The drawing under review shows one solid part. Ordinate dimensions are in mm from its lowest x, y, z. A direction names the side the tool comes from. Give positions to 0.01 mm unless a question says otherwise; leave off trailing zeros. Loops run counter-clockwise (first coordinate to the right, second up) from the corner with the lowest first, then second, coordinate; pieces in that order, holes last. Notation, with made-up numbers: M -38.75,59.25 L -4.75,59.25 A27 cw -4.75,91.25 Z; hole C 79,67 d10. An arc over 180 degrees is marked long. Put each result on its own line as item: value. Start each with the question number.
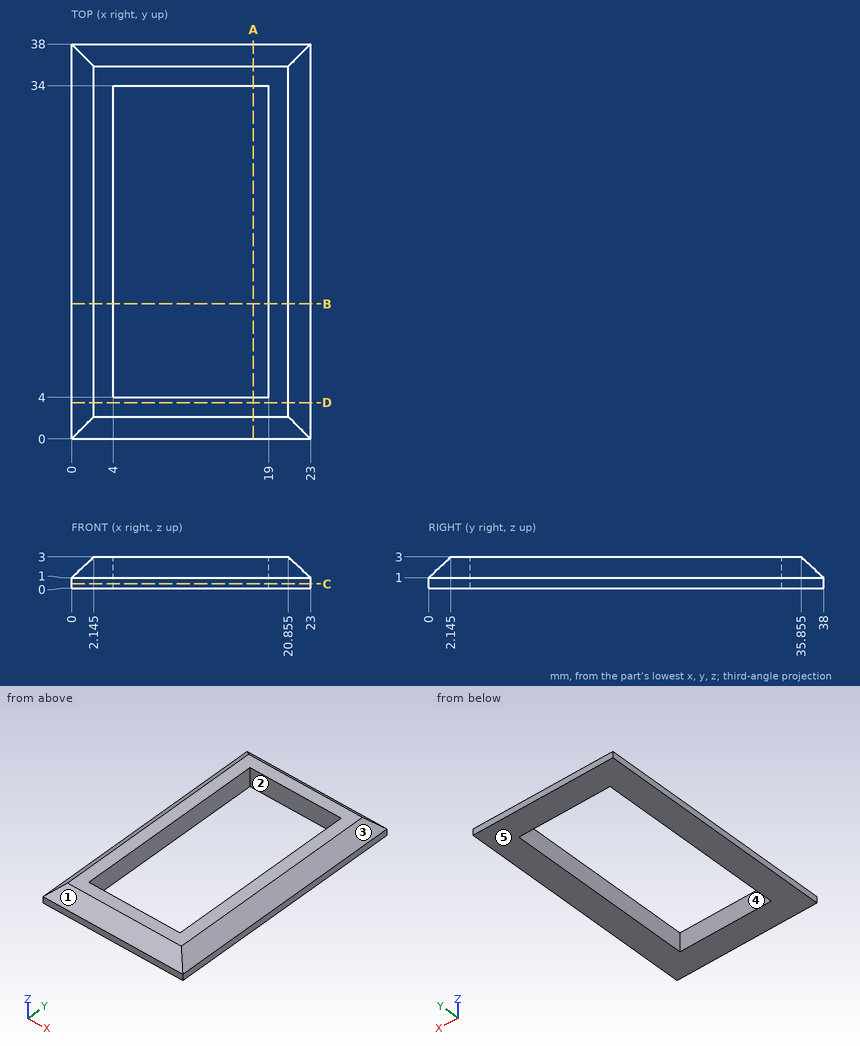
Item 1: Tool access review of the marked faces 1 and 2: name each direction out of +Z, -Z, +X, -X, +Y, -Y from which nothing blocks a thin tool from reaching the whole face with its end or side.
Item 2: Consider section A-A, the plane x = 17.5. Write out the cut boundary in (y, z) (1 decimal).
Item 3: Consider section D-D, the plane y = 3.5. Write out the cut boundary in (x, z) (1 decimal), plus the area to 3 significant figures.
Item 4: Consider section B-B, the plane y = 13. Write out the cut boundary in (x, z) (1 decimal), plus the area to 3 significant figures.
Item 5: Consider section C-C, the plane z = 0.4. Write out the cut boundary in (x, y).
Item 6: Draft analysis for pull direction X (two halves, no side actions). For the marked faces 3, 4 and 5, state which applies: +X half, -X half, draft (parallel to the pull), parting line (faces both ways), or undercut.
Item 7: To check wall thickness, follow L1, parallel to Y at x = 12.25, z = 0.35; L2, parallel to X at y = 5, z = 0.8; L3, parallel to Y at x = 15.25, z = 2.95. State the ranges of each line that lie inside material, in increasing order. Write a range as [from, to].
Item 8: Clearance check with flat-ended pins moving along their axes: pin 1 Ø1 at (x, z) = (8, 2) entering from -Y; pin 2 Ø1.5 at (x, z) = (15, 2) entering from -Y. State where each tip first meets the part, or that it passes through.
Report:
1. face 1: +Z, +X, -X, -Y
1. face 2: +Z, -Z
2. outline: M 0,0 L 4,0 L 4,3 L 2.1,3 L 0,1 Z; M 34,0 L 38,0 L 38,1 L 35.9,3 L 34,3 Z
3. outline: M 0,0 L 23,0 L 23,1 L 20.9,3 L 2.1,3 L 0,1 Z
3. area: 64.7 mm²
4. outline: M 0,0 L 4,0 L 4,3 L 2.1,3 L 0,1 Z; M 19,0 L 23,0 L 23,1 L 20.9,3 L 19,3 Z
4. area: 19.7 mm²
5. outline: M 0,0 L 23,0 L 23,38 L 0,38 Z; hole M 4,4 L 19,4 L 19,34 L 4,34 Z
6. face 3: +X half
6. face 4: undercut
6. face 5: draft
7. L1: [0, 4], [34, 38]
7. L2: [0, 4], [19, 23]
7. L3: [2.09, 4], [34, 35.91]
8. pin 1: y = 0.54
8. pin 2: y = 0.27
